Design review of the part shown in the three views and the two pictorial views. Dimensions are in mm from the part's minimum x, y and z. A direction names the side the tool comes from. Give positions to 0.01 mm unless a question says otherwise; leave off trailing zeros. Write each loop counter-clockwise with the first axis right and the second up, starting at its lowest first coordinate (ties: lowest second). Pieces come first, ordered by that corner, then holes. Notation, with made-up numbers: M 37,86.5 L 72,86.5 A9 cw 72,101.5 Z; hole C 85,-24 d1. An arc over 180 degrees is marked long. Use one line per item in the form item = value. Start each with the question number.
Q1. For probe 1 along Z at (x, y) = (14, 3.5); probe 2 along Z at (x, y) = (21.5, 5.25); probe 3 along Y at (x, z) = (8, 24), list the stretches that pass through material, from the lowest coordinate up. Write a range as [from, to].
Q2. Mouldability with a two-part tool opening along Z and no side actions: class the marked faces 1, 2 and 3 as released by +Z, released by -Z, zero draft, split by the parting line, or undercut.
Q3. Consider section D-D on z = 26.5. Write out the cut boundary in (x, y).
Q4. Consider section C-C on z = 19.5. Write out the cut boundary in (x, y).
Q5. Consider section A-A on x = 21. Write out the cut boundary in (y, z).
Q6. Tool access review of the marked faces 4 and 5: name each direction out of +Z, -Z, +X, -X, +Y, -Y from which nothing blocks a thin tool from reaching the whole face with its end or side.
Q7. Consider section B-B on y = 5. Write out the cut boundary in (x, z).
Q8. Clearance check with flat-ended pins moving along their axes: pin 1 Ø3 at (y, z) = (4.5, 17) entering from +X; pin 2 Ø1 at (x, z) = (1, 13) entering from -Y; pin 3 Ø1 at (x, y) = (21.5, 5) entering from +Z. State where each tip first meets the part, or that it passes through.
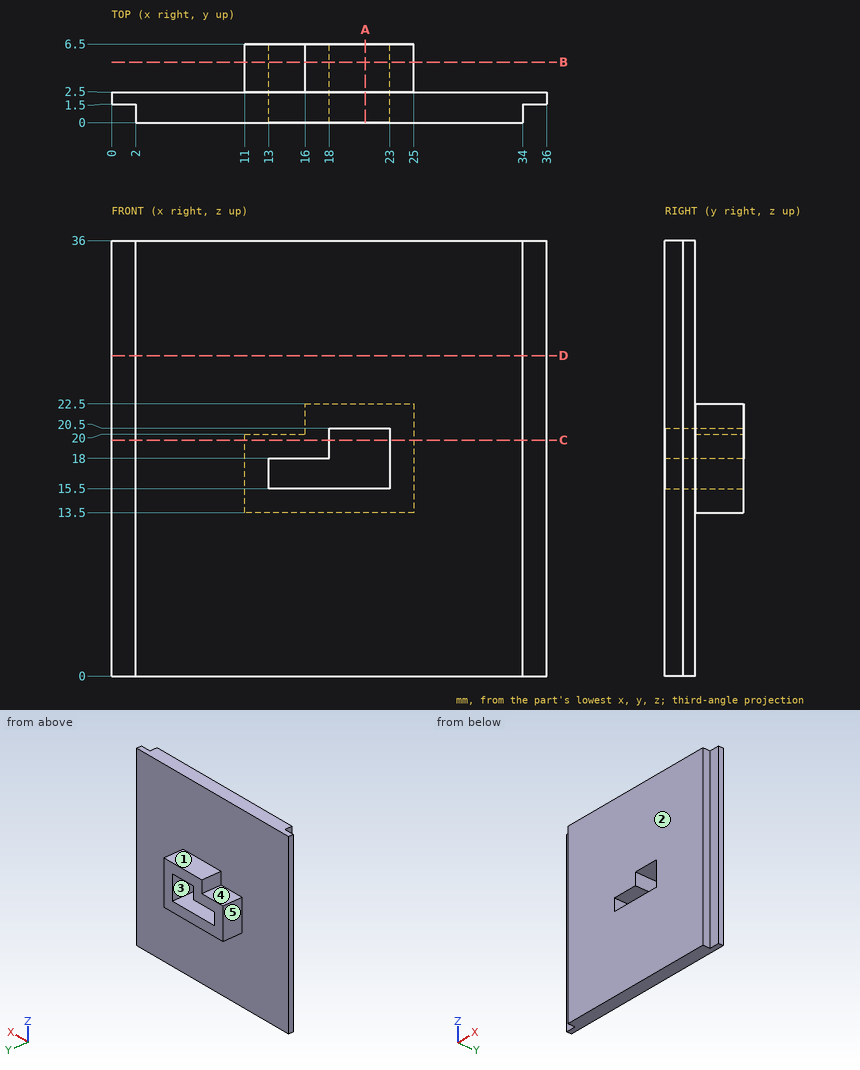
Working result:
q1.probe_1 = [13.5, 15.5], [18, 20]
q1.probe_2 = [13.5, 15.5], [20.5, 22.5]
q1.probe_3 = [0, 2.5]
q2.face_1 = released by +Z
q2.face_2 = zero draft
q2.face_3 = undercut
q3.outline = M 0,1.5 L 2,1.5 L 2,0 L 34,0 L 34,1.5 L 36,1.5 L 36,2.5 L 0,2.5 Z
q4.outline = M 0,1.5 L 2,1.5 L 2,0 L 18,0 L 18,6.5 L 11,6.5 L 11,2.5 L 0,2.5 Z; M 23,0 L 34,0 L 34,1.5 L 36,1.5 L 36,2.5 L 25,2.5 L 25,6.5 L 23,6.5 Z
q5.outline = M 0,0 L 2.5,0 L 2.5,13.5 L 6.5,13.5 L 6.5,15.5 L 0,15.5 Z; M 0,20.5 L 6.5,20.5 L 6.5,22.5 L 2.5,22.5 L 2.5,36 L 0,36 Z
q6.face_4 = +Z, -X, +Y
q6.face_5 = +Z, -Z, -X, +Y
q7.outline = M 11,13.5 L 25,13.5 L 25,22.5 L 16,22.5 L 16,20 L 11,20 Z; hole M 13,15.5 L 23,15.5 L 23,20.5 L 18,20.5 L 18,18 L 13,18 Z
q8.pin_1 = 25
q8.pin_2 = 1.5
q8.pin_3 = 22.5
